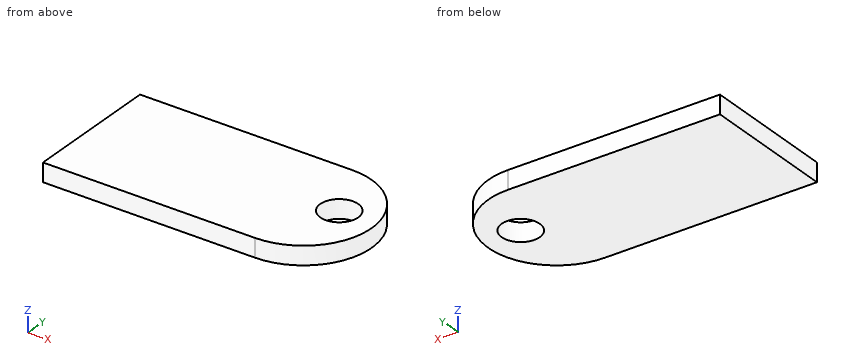
```python
from build123d import *

# Parameters (mm, degrees)
F1_DEPTH = 3.81
F2_R     = 3.897648
F3_DEPTH = 25.4


with BuildPart() as f1:
    # F0 (on Top) → F1 (new body)
    with BuildSketch(Plane.XY):
        with BuildLine():
            Line((-43.509971, 0), (0, 0))
            ThreePointArc((0, 0), (13.959449, 13.959449), (0, 27.918898))
            Line((0, 27.918898), (-43.509971, 27.918898))
            Line((-43.509971, 27.918898), (-43.509971, 0))
        make_face()
    extrude(amount=F1_DEPTH)

    # F2 (on face) → F3 (cut)
    with BuildSketch(Plane.XY.offset(3.81)):
        with Locations((6.163907, 15.591073)):
            Circle(F2_R)
    extrude(amount=-F3_DEPTH, mode=Mode.SUBTRACT)


solid = f1.part
```
For this review, take the finished solid that the model builds, in its own axes (mm). Round coordinates to 2 decimals unless told otherwise and drop trailing zeros. Order: outer loops, then holes, each group sorted by start corner. A loop starts at its lowest first (then second) coordinate and runs counter-clockwise, first axis right, second up. Notation, with made-up numbers: (27, -24) -> (47, -24) arc R24 ccw to (47, -6) -> close; hole circle Ø3 at (61.25, 22.25). An arc over 180 degrees is marked (long way). Use a Markdown table: item, result.
Item 1: Take a section at D-D (y = 6.75). State the section outline as (x, z) points, plus the area to 3 significant figures.
Resolved:
| item | result |
|---|---|
| outline | (-43.51, 0) -> (11.95, 0) -> (11.95, 3.81) -> (-43.51, 3.81) -> close |
| area | 211 mm² |
Item 2: For line 1 along X through (y, z) = (15, 3.6); line 2 along X through (y, z) = (12.75, 2.65); line 3 along Y through (x, z) = (8, 1.2), list the stretches that pass through material, from the lowest coordinate up. Write a range as [from, to].
Resolved:
| item | result |
|---|---|
| line 1 | x = [-43.51, 2.31], [10.02, 13.92] |
| line 2 | x = [-43.51, 3.5], [8.83, 13.91] |
| line 3 | y = [2.52, 12.15], [19.03, 25.4] |
Item 3: Take a section at C-C (y = 13.5). State the section outline as (x, z) points, plus the area to 3 significant figures.
Resolved:
| item | result |
|---|---|
| outline | (-43.51, 0) -> (2.87, 0) -> (2.87, 3.81) -> (-43.51, 3.81) -> close; (9.45, 0) -> (13.95, 0) -> (13.95, 3.81) -> (9.45, 3.81) -> close |
| area | 194 mm² |
Item 4: Take a section at A-A (y = 16.5). State the section outline as (x, z) points.
Resolved:
| item | result |
|---|---|
| outline | (-43.51, 0) -> (2.37, 0) -> (2.37, 3.81) -> (-43.51, 3.81) -> close; (9.95, 0) -> (13.73, 0) -> (13.73, 3.81) -> (9.95, 3.81) -> close |
Item 5: Take a section at B-B (z = 2.75). State the section outline as (x, y) points.
Resolved:
| item | result |
|---|---|
| outline | (-43.51, 0) -> (0, 0) arc R13.96 ccw to (0, 27.92) -> (-43.51, 27.92) -> close; hole circle Ø7.8 at (6.16, 15.59) |
